Geometry: final body of the model. Coordinates: model frame, mm. Give positions to 0.01 mm unless a question says otherwise; leave off trailing zeros. Order: outer loops, then holes, each group sorted by start corner. A loop starts at its lowest first (then second) coordinate and runs counter-clockwise, first axis right, second up. Notation, with made-up numbers: M 36,13 L 79,13 A7 cw 79,17 Z; hole C 73,57 d5. An arc over 180 degrees is marked long. Use CSV: the item, a comma, the result in double quotes.
```python
from build123d import *

# Parameters (mm, degrees)
SKETCH1_R           = 3.55
BOSS_EXTRUDE1_DEPTH = 7
SKETCH2_R           = 3.1
CUT_EXTRUDE1_DEPTH  = 6.5
FILLET1_R           = 0.2
FILLET2_R           = 1


with BuildPart() as part:
    # Sketch1 → Boss-Extrude1 (new body)
    with BuildSketch(Plane.XY):
        Circle(SKETCH1_R)
    extrude(amount=BOSS_EXTRUDE1_DEPTH)

    # Sketch2 → Cut-Extrude1 (cut)
    with BuildSketch(Plane.XY.offset(7)):
        Circle(SKETCH2_R)
    extrude(amount=-CUT_EXTRUDE1_DEPTH, mode=Mode.SUBTRACT)

    # Fillet1
    fillet1_edges = [part.edges().sort_by_distance(p)[0] for p in [
        (-3.55, 0, 7),
        (-3.1, 0, 7),
    ]]
    fillet(fillet1_edges, radius=FILLET1_R)

    # Fillet2
    fillet2_edges = [part.edges().sort_by_distance(p)[0] for p in [
        (-3.55, 0, 0),
    ]]
    fillet(fillet2_edges, radius=FILLET2_R)


solid = part.part
```
1. Section A-A, the plane y = 0. Return the cut outline in (x, z).
Answer:
outline,"M -3.55,1 A1 ccw -2.55,0 L 2.55,0 A1 ccw 3.55,1 L 3.55,6.8 A0.2 ccw 3.35,7 L 3.3,7 A0.2 ccw 3.1,6.8 L 3.1,0.5 L -3.1,0.5 L -3.1,6.8 A0.2 ccw -3.3,7 L -3.35,7 A0.2 ccw -3.55,6.8 Z"
2. Pull-direction query (X, two-part tool) for faces 1 (the face through (0, 0, 0.5)), 2 (the face through (-0.46, 3.52, 3.86)), 3 (the face through (0, 0, 0)); classes: +X half, -X half, draft (parallel to the pull), parting line (faces both ways), or undercut.
Answer:
face 1,"undercut"
face 2,"parting line"
face 3,"draft"
3. Pin query (flat end, axial travel): pin 1 Ø1.9 at (x, y) = (-1, -1) entering from +Z; pin 2 Ø1 at (y, z) = (1.5, 4) entering from -X; pin 3 Ø4 at (y, z) = (-2.5, 6) entering from -X. Return the tip coordinate at first contact, or that it passes through.
Answer:
pin 1,"z = 0.5"
pin 2,"x = -3.41"
pin 3,"x = -3.51"
4. Section B-B, the plane z = 5.25. Return the cut outline in (x, y), plus the area to 3 significant figures.
Answer:
outline,"C 0,0 d7.1; hole C 0,0 d6.2"
area,"9.40 mm2"
5. Line query: line 1 (Y direction, x = 0, z = 2.25); line 2 (Z direction, x = -2.25, y = 0); line 3 (X direction, y = 1.75, z = 4). Output: solid intervals per line, ascending.
Answer:
line 1,"-3.55 to -3.1, 3.1 to 3.55"
line 2,"0 to 0.5"
line 3,"-3.09 to -2.56, 2.56 to 3.09"
